from build123d import *
from build123d.topology import SkipClean

# Parameters (mm, degrees)
SKETCH1_R              = 9.5
BOSS_EXTRUDE1_DEPTH    = 48
SKETCH2_W              = 34
SKETCH2_H              = 30
CUT_EXTRUDE1_DEPTH     = 62.481704596
BOSS_EXTRUDE2_START    = -2.5
SKETCH3_R              = 9.5
SKETCH3_R_2            = 2.4
BOSS_EXTRUDE2_DEPTH    = 2.5
SKETCH4_R              = 9.5
SKETCH4_R_2            = 4.2
BOSS_EXTRUDE3_DEPTH    = 7
SKETCH5_R              = 4.2
BOSS_EXTRUDE4_DEPTH    = 11
BOSS_EXTRUDE5_DEPTH    = 48
CUT_EXTRUDE2_START     = -48
CUT_EXTRUDE2_OUTLINE_R = 2.65
CUT_EXTRUDE2_DEPTH     = 48
CUT_EXTRUDE3_START     = -4.5
SKETCH8_R              = 9.5
CUT_EXTRUDE3_DEPTH     = 4.5
SKETCH9_R              = 6.067807638
CUT_EXTRUDE4_DEPTH     = 4.5
SKETCH10_R             = 9.5
BOSS_EXTRUDE6_DEPTH    = 4.5
SKETCH11_R             = 4.2
BOSS_EXTRUDE7_DEPTH    = 3.5
SKETCH12_R             = 2.4
BOSS_EXTRUDE8_DEPTH    = 2.5
SKETCH13_W             = 35
SKETCH13_H             = 34
CUT_EXTRUDE5_DEPTH     = 14.5
SKETCH15_R             = 3.436413098
BOSS_EXTRUDE9_DEPTH    = 10
BOSS_EXTRUDE10_DEPTH   = 0.5
SKETCH18_R             = 4.2
CUT_EXTRUDE8_DEPTH     = 0.5
CUT_EXTRUDE9_DEPTH     = 69.529190861
BOSS_EXTRUDE11_DEPTH   = 7
CUT_EXTRUDE10_DEPTH    = 80.22909819
BOSS_EXTRUDE12_DEPTH   = 41.5
SKETCH25_R             = 4.2
CUT_EXTRUDE11_DEPTH    = 0.5


# Read off the part's stored shape, not the designer's step: Cut-Extrude2
with BuildPart() as part:
    # Sketch1 → Boss-Extrude1 (new body)
    with BuildSketch(Plane.XY):
        with BuildLine():
            Line((-12, 0), (-12, 30))
            Line((-12, 30), (12, 30))
            Line((12, 30), (12, 0))
            ThreePointArc((12, 0), (0, -12), (-12, 0))
        make_face()
        Circle(SKETCH1_R, mode=Mode.SUBTRACT)
    extrude(amount=-BOSS_EXTRUDE1_DEPTH)

    # Sketch2 → Cut-Extrude1 (cut, through all)
    with BuildSketch(Plane.ZY.offset(12)):
        with Locations((-24, 3)):
            Rectangle(SKETCH2_W, SKETCH2_H)
    extrude(amount=-CUT_EXTRUDE1_DEPTH, mode=Mode.SUBTRACT)

    # Sketch3 → Boss-Extrude2 (add)
    with BuildSketch(Plane(origin=(0, 0, -48), x_dir=(-1, 0, 0), z_dir=(0, 0, -1)).offset(BOSS_EXTRUDE2_START)):
        Circle(SKETCH3_R)
        Circle(SKETCH3_R_2, mode=Mode.SUBTRACT)
    extrude(amount=BOSS_EXTRUDE2_DEPTH)

    # Sketch4 → Boss-Extrude3 (add)
    with BuildSketch(Plane.XY):
        with Locations(Location((0, 0, 0), (0, 0, 180))):
            Circle(SKETCH4_R)
        Circle(SKETCH4_R_2, mode=Mode.SUBTRACT)
    extrude(amount=-BOSS_EXTRUDE3_DEPTH)

    # Sketch5 → Boss-Extrude4 (add)
    with BuildSketch(Plane.XY):
        Circle(SKETCH5_R)
    extrude(amount=-BOSS_EXTRUDE4_DEPTH)

    # Sketch6 → Boss-Extrude5 (add)
    with BuildSketch(Plane(origin=(0, 0, -48), x_dir=(-1, 0, 0), z_dir=(0, 0, -1))):
        Polygon((12, 30), (12, 18), (18, 18), (38, 18), (38, 30), align=None)
    extrude(amount=-BOSS_EXTRUDE5_DEPTH)

    # Cut-Extrude2 outline → Cut-Extrude2 (cut)
    with BuildSketch(Plane.XY.offset(CUT_EXTRUDE2_START)):
        Circle(CUT_EXTRUDE2_OUTLINE_R)
    extrude(amount=CUT_EXTRUDE2_DEPTH, mode=Mode.SUBTRACT)

    # Sketch8 → Cut-Extrude3 (cut)
    with BuildSketch(Plane(origin=(0, 0, -7), x_dir=(-1, 0, 0), z_dir=(0, 0, -1)).offset(CUT_EXTRUDE3_START)):
        Circle(SKETCH8_R)
    extrude(amount=CUT_EXTRUDE3_DEPTH, mode=Mode.SUBTRACT)


with BuildPart() as cut_extrude3_piece_1:
    # of the separate pieces the step leaves, piece 1, a body of its own (cut_extrude3_pieces)
    add(part.part.solids().sort_by_distance((-12, 0, 0))[0])

    # Sketch10 → Boss-Extrude6 (add)
    with BuildSketch(Plane.XY.offset(-45.5)):
        with Locations(Location((0, 0, 0), (0, 0, 90))):
            Circle(SKETCH10_R)
    extrude(amount=BOSS_EXTRUDE6_DEPTH)

    # Sketch11 → Boss-Extrude7 (add)
    with BuildSketch(Plane.XY.offset(-41)):
        with Locations(Location((0, 0, 0), (0, 0, 180))):
            Circle(SKETCH11_R)
    extrude(amount=BOSS_EXTRUDE7_DEPTH)

    # Sketch12 → Boss-Extrude8 (add)
    with BuildSketch(Plane(origin=(0, 0, -48), x_dir=(-1, 0, 0), z_dir=(0, 0, -1))):
        Circle(SKETCH12_R)
    extrude(amount=-BOSS_EXTRUDE8_DEPTH)

    # Sketch13 → Cut-Extrude5 (cut)
    with BuildSketch(Plane(origin=(0, 30, 0), x_dir=(1, 0, 0), z_dir=(0, 1, 0))):
        with Locations((-5.5, 24)):
            Rectangle(SKETCH13_W, SKETCH13_H)
    extrude(amount=-CUT_EXTRUDE5_DEPTH, mode=Mode.SUBTRACT)

    # Sketch15 → Boss-Extrude9 (add)
    with BuildSketch(Plane(origin=(0, 0, -48), x_dir=(-1, 0, 0), z_dir=(0, 0, -1))):
        Circle(SKETCH15_R)
    extrude(amount=-BOSS_EXTRUDE9_DEPTH)

    # Sketch16 → Boss-Extrude10 (add)
    with SkipClean():  # the faces are left unmerged after this step: merging them gives an invalid solid
        with BuildSketch(Plane(origin=(0, 0, -48), x_dir=(-1, 0, 0), z_dir=(0, 0, -1))):
            Polygon((38, 30), (-12, 30), (-12, 18), (12, 18), (38, 18), align=None)
            with BuildLine():
                Line((-12, 0), (12, 0))
                ThreePointArc((12, 0), (0, -12), (-12, 0))
            make_face()
            with BuildLine():
                ThreePointArc((12, 0), (0, 12), (-12, 0))
                Line((-12, 0), (12, 0))
            make_face()
            with BuildLine():
                Line((12, 0), (-12, 0))
                ThreePointArc((-12, 0), (0, -12), (12, 0))
            make_face()
            with BuildLine():
                Line((12, 18), (-12, 18))
                Line((-12, 18), (-12, 0))
                ThreePointArc((-12, 0), (0, 12), (12, 0))
                Line((12, 0), (12, 18))
            make_face()
        extrude(amount=BOSS_EXTRUDE10_DEPTH)

    # Sketch18 → Cut-Extrude8 (cut)
    with SkipClean():  # the faces are left unmerged after this step: merging them gives an invalid solid
        with BuildSketch(Plane.XY.offset(-41)):
            with BuildLine():
                Line((12, 30), (-23, 30))
                Line((-23, 30), (-23, 18))
                Line((-23, 18), (-12, 18))
                Line((-12, 18), (-12, 0))
                ThreePointArc((-12, 0), (0, -12), (12, 0))
                Line((12, 0), (12, 30))
            make_face()
            Circle(SKETCH18_R, mode=Mode.SUBTRACT)
        extrude(amount=-CUT_EXTRUDE8_DEPTH, mode=Mode.SUBTRACT)

    # Sketch19 → Cut-Extrude9 (cut, through all)
    with SkipClean():  # the faces are left unmerged after this step: merging them gives an invalid solid
        with BuildSketch(Plane.XY):
            with BuildLine():
                ThreePointArc((11, 0), (0, -11), (-11, 0))
                Line((-11, 0), (-12, 0))
                ThreePointArc((-12, 0), (0, -12), (12, 0))
                Line((12, 0), (12, 30))
                Line((12, 30), (11, 30))
                Line((11, 30), (11, 0))
            make_face()
        extrude(amount=-CUT_EXTRUDE9_DEPTH, mode=Mode.SUBTRACT)

    # Sketch21 → Boss-Extrude11 (add)
    with SkipClean():  # the faces are left unmerged after this step: merging them gives an invalid solid
        with BuildSketch(Plane.XY):
            with BuildLine():
                Line((-55, -11), (0, -11))
                ThreePointArc((0, -11), (-7.778174593, -7.778174593), (-11, 0))
                Line((-11, 0), (-12, 0))
                Line((-12, 0), (-12, 18))
                Line((-12, 18), (-29.285566016, 18))
                ThreePointArc((-29.285566016, 18), (-44.085437149, 5.222560402), (-55, -11))
            make_face()
        boss_extrude11 = extrude(amount=-BOSS_EXTRUDE11_DEPTH)

    # Mirror2: Boss-Extrude11 across plane
    with SkipClean():  # the faces are left unmerged after this step: merging them gives an invalid solid
        add(boss_extrude11.mirror(Plane.XY.offset(-24.25)))

    # Sketch23 → Cut-Extrude10 (cut, through all)
    with SkipClean():  # the faces are left unmerged after this step: merging them gives an invalid solid
        with BuildSketch(Plane.XY):
            with BuildLine():
                Line((11, 30), (-38, 30))
                Line((-38, 30), (-38, 11.325220695))
                ThreePointArc((-38, 11.325220695), (-15.219016868, 25.173069355), (11, 30))
            make_face()
        extrude(amount=-CUT_EXTRUDE10_DEPTH, mode=Mode.SUBTRACT)

    # Sketch24 → Boss-Extrude12 (add)
    with SkipClean():  # the faces are left unmerged after this step: merging them gives an invalid solid
        with BuildSketch(Plane.XY):
            with BuildLine():
                ThreePointArc((-23, 21.6788275), (-41.60205739, 7.887419381), (-55, -11))
                Line((-55, -11), (-51.635998377, -11))
                ThreePointArc((-51.635998377, -11), (-39.486754135, 5.75970176), (-23, 18.276837089))
                Line((-23, 18.276837089), (-23, 21.6788275))
            make_face()
        extrude(amount=-BOSS_EXTRUDE12_DEPTH)

    # Sketch25 → Cut-Extrude11 (cut)
    # profile 1 of 3: a face of its own
    with BuildSketch(Plane.XY.offset(-41.5)):
        with BuildLine():
            ThreePointArc((11, 27), (-6.550595226, 24.784456384), (-23, 18.276837089))
            Line((-23, 18.276837089), (-23, 18))
            Line((-23, 18), (-23.499204657, 18))
            ThreePointArc((-23.499204657, 18), (-39.685914386, 5.555259732), (-51.635998377, -11))
            Line((-51.635998377, -11), (0, -11))
            ThreePointArc((0, -11), (-7.778174593, 7.778174593), (11, 0))
            Line((11, 0), (11, 27))
        make_face()
    # profile 2 of 3: a face of its own
    with BuildSketch(Plane.XY.offset(-41.5)):
        with BuildLine():
            ThreePointArc((0, -11), (7.778174593, -7.778174593), (11, 0))
            ThreePointArc((11, 0), (-7.778174593, 7.778174593), (0, -11))
        make_face()
        Circle(SKETCH25_R, mode=Mode.SUBTRACT)
    # profile 3 of 3: a face of its own
    with BuildSketch(Plane.XY.offset(-41.5)):
        with BuildLine():
            ThreePointArc((11, 30), (-6.501727856, 27.889455027), (-23, 21.6788275))
            Line((-23, 21.6788275), (-23, 18.276837089))
            ThreePointArc((-23, 18.276837089), (-6.550595226, 24.784456384), (11, 27))
            Line((11, 27), (11, 30))
        make_face()
    extrude(amount=-CUT_EXTRUDE11_DEPTH, mode=Mode.SUBTRACT)


with BuildPart() as cut_extrude3_piece_2:
    # of the separate pieces the step leaves, piece 2, a body of its own (cut_extrude3_pieces)
    add(part.part.solids().sort_by_distance((4.2, 0, -7))[0])

    # Sketch9 → Cut-Extrude4 (cut)
    with BuildSketch(Plane(origin=(0, 0, -11), x_dir=(-1, 0, 0), z_dir=(0, 0, -1))):
        Circle(SKETCH9_R)
    extrude(amount=-CUT_EXTRUDE4_DEPTH, mode=Mode.SUBTRACT)


solid = cut_extrude3_piece_1.part
Can you work these out from the model? Positions are in its coordinate system, mm. A direction names the side the tool comes from. Coordinates: 2 decimals unless noted, no trailing zeros. Loops run counter-clockwise (first coordinate to the right, second up) from the corner with the lowest first, then second, coordinate; pieces in that order, holes last. Notation, with made-up numbers: (-11, 89) - (-2, 89) arc R18 ccw to (-2, 119) - close; hole circle Ø4 at (-11, -29.5). An arc over 180 degrees is marked (long way). Answer as a JSON object with one key per item and string values. Group by question number.
Item 1: If we mould it in two halves opening along X, with no side actions, what happens to faces 4 (the face through (-14, 5, -42)), 5 (the face through (2.45, -1.01, -1.27)), 6 (the face through (-32, -11, -6)), 7 (the face through (7.863, -7.692, -3.451))? For each: released by +X, released by -X, zero draft, split by the parting line, or undercut.
Item 2: If I drill on L1, parallel to Z at x = 1.5, y = 18.5; L2, parallel to Z at x = -6, y = 2.5; L3, parallel to Y at x = 0, z = -1, over which ranges is the centre line in solid material (lowest first)? Write a range as from..to.
Item 3: If we section it at A-A (x = -11.5): List the corners of the cut face in (y, z) for me.
Item 4: On a 3-axis mill with a long thin cutter (end or side, diameter ignored), from which of +Z, -Z, +X, -X, +Y, -Y can I reach the whole of each face in a straight line? I mean faces 1 (the face through (-4.38, -8.43, -4.72)), 2 (the face through (-14, 10, -7)), 3 (the face through (-23, 20, -24)). Say none if no direction works.
Item 5: If we section it at B-B (x = 1.5): List the corners of the cut face in (y, z) for me, plus the area to 3 significant figures.
Item 6: If we section it at D-D (y = -5.5): List the corners of the cut face in (x, z) for me.
Item 7: If we section it at C-C (z = -45.5): List the corners of the cut face in (x, y) for me.
Item 8: For pin 1 (4 mm diameter, centred on x = -0.5, y = 0.5, fed in from +Z); pin 2 (1.1 mm diameter, centred on y = 19, z = -29.5, fed in from +X); pin 3 (1.5 mm diameter, centred on x = -7.5, z = -8, fed in from +Y); pin 4 (3 mm diameter, centred on y = -0.5, z = -32.5, fed in from -X), each with a flat end and sliding along its axis, tell me the tip position at first contact or that it passes through.
Returned:
{
 "1": {"face 4": "undercut", "face 5": "undercut", "face 6": "zero draft", "face 7": "released by +X"},
 "2": {"L1": "z = -48.5..-42, -7..0", "L2": "z = -48.5..-42, -2.5..0", "L3": "y = -11..-2.65, 2.65..29.17"},
 "3": {"outline": "(-11, -48.5) - (26.48, -48.5) - (26.48, -42) - (-11, -42) - close; (-11, -7) - (26.48, -7) - (26.48, 0) - (-11, 0) - close"},
 "4": {"face 1": "none", "face 2": "+X, -Y", "face 3": "+X, +Y, -Y"},
 "5": {"outline": "(-10.9, -48.5) - (29.38, -48.5) - (29.38, -42) - (3.92, -42) - (3.92, -37.5) - (-3.92, -37.5) - (-3.92, -42) - (-10.9, -42) - close; (-10.9, -7) - (-9.38, -7) - (-9.38, -2.5) - (-2.18, -2.5) - (-2.18, 0) - (-10.9, 0) - close; (2.18, -2.5) - (9.38, -2.5) - (9.38, -7) - (29.38, -7) - (29.38, 0) - (2.18, 0) - close", "area": "484 mm²"},
 "6": {"outline": "(-51.98, -48.5) - (9.53, -48.5) - (9.53, -42) - (-48.45, -42) - (-48.45, -7) - (-7.75, -7) - (-7.75, -2.5) - (7.75, -2.5) - (7.75, -7) - (9.53, -7) - (9.53, 0) - (-51.98, 0) - close"},
 "7": {"outline": "(-55, -11) - (0, -11) arc R11 ccw to (11, 0) - (11, 30) arc R73.62 ccw to start"},
 "8": {"pin 1": "stops at z = 0", "pin 2": "stops at x = -23", "pin 3": "passes through", "pin 4": "stops at x = -49.73"}
}
